Part model, mm, in its own coordinate system. A direction names the side the tool comes from. Coordinates: 2 decimals unless noted, no trailing zeros. Loops run counter-clockwise (first coordinate to the right, second up) from the corner with the lowest first, then second, coordinate; pieces in that order, holes last. Notation, with made-up numbers: (29.5, 54.25) -> (52.5, 54.25) arc R16 ccw to (52.5, 60.25) -> close; hole circle Ø2 at (-29.75, 16.25). An arc over 180 degrees is marked (long way). Use one line per item in the form item = value. Start each with the question number.
(1) Band-saw the part on B-B on z = 1.5. Give the cut face in (x, y).
(2) Drill centre lines: L1, parallel to Y at x = 10.25, z = 8.75; L2, parallel to Y at x = 12.5, z = 10.25; L3, parallel to Z at x = -10.5, y = 4. Where is each one in solid material? Low to high. Write a range as [from, to].
(3) Band-saw the part on A-A on x = 12.75. Give the cut face in (y, z), then the cut area to 3 significant figures.
(4) Mould opens along Y. For faces 1 (the flat face through (-9, 30, 3)), 2 (the flat face through (-12, 10, 14)), 3 (the cylindrical face through (0.1, -23.5, 5.6)), 4 (the flat face through (0, 7, 16)) say: +Y half, -Y half, draft (parallel to the pull), parting line (faces both ways), or undercut.
(5) Band-saw the part on D-D on x = 0. Give the cut face in (y, z), then the cut area to 4 significant figures.
(6) Band-saw the part on C-C on y = -5. Give the cut face in (x, z), then the cut area to 3 significant figures.
(7) 3-axis set-ups, long thin cutter, end or side, ignore diameter. For faces 5 (the flat face through (0, -16, 13)), 6 (the flat face through (-12, 2, 11)), 7 (the flat face through (-9, 27, 10)): which of +Z, -Z, +X, -X, +Y, -Y reach the whole face in a straight line?
(8) Pin check, flat tips, straight feed: P1, Ø2, axis at x = -2.5, z = 10, coming from the -Y side; P2, Ø11, axis at x = -7, y = -22.5, coming from the +Z side; P3, Ø5, axis at y = 3.5, z = 11.5, coming from the +X side. Stop position of each tip, or through.
```python
from build123d import *

# Parameters (mm, degrees)
SKETCH_1_W          = 30
SKETCH_1_H          = 60
EXTRUDE_1_DEPTH     = 16
SKETCH_2_W          = 4
SKETCH_2_H          = 5
SKETCH_2_W_2        = 5
SKETCH_2_H_2        = 14
CUT_EXTRUDE_1_DEPTH = 46.343136195
SKETCH_3_R          = 6.5
SKETCH_3_W          = 6
SKETCH_3_H          = 5
CUT_EXTRUDE_2_DEPTH = 38.161808352
SKETCH_4_W          = 5
SKETCH_4_H          = 17
CUT_EXTRUDE_3_DEPTH = 38.161808352
SKETCH_5_W          = 7
SKETCH_5_H          = 17
CUT_EXTRUDE_4_DEPTH = 5
SKETCH_6_W          = 5
SKETCH_6_H          = 16
CUT_EXTRUDE_5_DEPTH = 7


with BuildPart() as part:
    # Эскиз1 → Бобышка-Вытянуть1 (new body)
    with BuildSketch(Plane.XY):
        Rectangle(SKETCH_1_W, SKETCH_1_H)
    extrude(amount=EXTRUDE_1_DEPTH)

    # Эскиз2 → Вырез-Вытянуть1 (cut, through all)
    with BuildSketch(Plane.ZY.offset(15)):
        with Locations((8, 27.5)):
            Rectangle(SKETCH_2_W, SKETCH_2_H)
        with Locations((13.5, -23)):
            Rectangle(SKETCH_2_W_2, SKETCH_2_H_2)
    extrude(amount=-CUT_EXTRUDE_1_DEPTH, mode=Mode.SUBTRACT)

    # Эскиз3 → Вырез-Вытянуть2 (cut, through all)
    with BuildSketch(Plane.XY.offset(16)):
        with Locations((0, -30)):
            Circle(SKETCH_3_R)
        with Locations((0, 27.5)):
            Rectangle(SKETCH_3_W, SKETCH_3_H)
    extrude(amount=-CUT_EXTRUDE_2_DEPTH, mode=Mode.SUBTRACT)

    # Эскиз4 → Вырез-Вытянуть3 (cut, through all)
    with BuildSketch(Plane.XY.offset(16)):
        with Locations((12.5, 1.5)):
            Rectangle(SKETCH_4_W, SKETCH_4_H)
    extrude(amount=-CUT_EXTRUDE_3_DEPTH, mode=Mode.SUBTRACT)

    # Эскиз5 → Вырез-Вытянуть4 (cut)
    with BuildSketch(Plane.XY.offset(16)):
        with Locations((-11.5, 1.5)):
            Rectangle(SKETCH_5_W, SKETCH_5_H)
    extrude(amount=-CUT_EXTRUDE_4_DEPTH, mode=Mode.SUBTRACT)

    # Эскиз6 → Вырез-Вытянуть5 (cut)
    with BuildSketch(Plane.XZ.offset(-10)):
        with Locations((12.5, 8)):
            Rectangle(SKETCH_6_W, SKETCH_6_H)
    extrude(amount=-CUT_EXTRUDE_5_DEPTH, mode=Mode.SUBTRACT)


solid = part.part
```
A:
q1.outline = (-15, -30) -> (-6.5, -30) arc R6.5 cw to (6.5, -30) -> (15, -30) -> (15, -7) -> (10, -7) -> (10, 17) -> (15, 17) -> (15, 30) -> (3, 30) -> (3, 25) -> (-3, 25) -> (-3, 30) -> (-15, 30) -> close
q2.L1 = [-30, -7], [17, 25]
q2.L2 = [-30, -7], [17, 30]
q2.L3 = [0, 11]
q3.outline = (-30, 0) -> (-7, 0) -> (-7, 16) -> (-16, 16) -> (-16, 11) -> (-30, 11) -> close; (17, 0) -> (30, 0) -> (30, 6) -> (25, 6) -> (25, 10) -> (30, 10) -> (30, 16) -> (17, 16) -> close
q3.area = 486 mm²
q4.face_1 = +Y half
q4.face_2 = undercut
q4.face_3 = -Y half
q4.face_4 = draft
q5.outline = (-23.5, 0) -> (25, 0) -> (25, 16) -> (-16, 16) -> (-16, 11) -> (-23.5, 11) -> close
q5.area = 738.5 mm²
q6.outline = (-15, 0) -> (10, 0) -> (10, 16) -> (-8, 16) -> (-8, 11) -> (-15, 11) -> close
q6.area = 365 mm²
q7.face_5 = +Z, +X, -X, -Y
q7.face_6 = +Z, -X
q7.face_7 = +X, -X, +Y
q8.P1 = -24.52
q8.P2 = 11
q8.P3 = 10
